```python
from build123d import *

# Parameters (mm, degrees)
SKETCH_1_W          = 20
SKETCH_1_H          = 20
SKETCH_1_R          = 1
EXTRUDE_1_DEPTH     = 28
EXTRUDE_2_DEPTH     = 1.6
SKETCH_3_R          = 2
EXTRUDE_3_DEPTH     = 10.4
CUT_EXTRUDE_START   = -7
CUT_EXTRUDE_4_DEPTH = 7


with BuildPart() as part:
    # 草图1 → 凸台-拉伸1 (new body)
    with BuildSketch(Plane(origin=(0, 0, 0), x_dir=(1, 0, 0), z_dir=(0, 1, 0))):
        with Locations((10, 10)):
            Rectangle(SKETCH_1_W, SKETCH_1_H)
        with Locations(Location((17.7, 2.3, 0), (0, 0, 270))):
            Circle(SKETCH_1_R, mode=Mode.SUBTRACT)
        with Locations(Location((17.7, 17.7, 0), (0, 0, 270))):
            Circle(SKETCH_1_R, mode=Mode.SUBTRACT)
        with Locations(Location((2.3, 17.7, 0), (0, 0, 270))):
            Circle(SKETCH_1_R, mode=Mode.SUBTRACT)
        with Locations(Location((2.3, 2.3, 0), (0, 0, 270))):
            Circle(SKETCH_1_R, mode=Mode.SUBTRACT)
    extrude(amount=EXTRUDE_1_DEPTH)

    # 草图2 → 凸台-拉伸2 (add)
    with BuildSketch(Plane(origin=(0, 28, 0), x_dir=(1, 0, 0), z_dir=(0, 1, 0))):
        with BuildLine():
            ThreePointArc((2, 10), (10, 2), (18, 10))
            Line((18, 10), (2, 10))
        make_face()
        with BuildLine():
            Line((2, 10), (18, 10))
            ThreePointArc((18, 10), (10, 18), (2, 10))
        make_face()
    extrude(amount=EXTRUDE_2_DEPTH)

    # 草图3 → 凸台-拉伸3 (add)
    with BuildSketch(Plane(origin=(0, 29.6, 0), x_dir=(1, 0, 0), z_dir=(0, 1, 0))):
        with Locations(Location((10, 10, 0), (0, 0, 270))):
            Circle(SKETCH_3_R)
    extrude(amount=EXTRUDE_3_DEPTH)

    # 草图4 → 切除-拉伸4 (cut)
    with BuildSketch(Plane(origin=(0, 40, 0), x_dir=(1, 0, 0), z_dir=(0, 1, 0)).offset(CUT_EXTRUDE_START)):
        with BuildLine():
            Line((11.501110762, 11.321615103), (11.501110762, 10))
            Line((11.501110762, 10), (11.501110762, 8.678384897))
            ThreePointArc((11.501110762, 8.678384897), (11.871125533, 9.293679083), (12, 10))
            ThreePointArc((12, 10), (11.871125533, 10.706320917), (11.501110762, 11.321615103))
        make_face()
    extrude(amount=CUT_EXTRUDE_4_DEPTH, mode=Mode.SUBTRACT)


solid = part.part
```
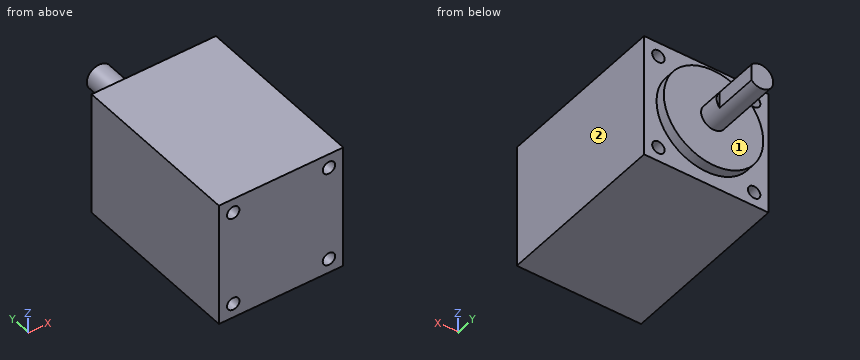
Check sheet for the modelled part. Datum: model origin and axes. Units: mm. Face numbers are marked on the shaded views. A direction names the side the tool comes from. Give positions to 0.01 mm unless a question says otherwise; leave off trailing zeros. Loops run counter-clockwise (first coordinate to the right, second up) from the corner with the lowest first, then second, coordinate; pieces in that order, holes last. Notation, with made-up numbers: M 31,41 L 90,41 A16 cw 90,47 Z; hole C -29,35 d4. An arc over 180 degrees is marked long. Answer in a Markdown table with one row per item.
1) Thickness scan on line 1 (X direction, y = 13, z = -17.7); line 2 (Y direction, x = 4.75, z = -13.5); line 3 (Y direction, x = 2.25, z = -5). Record the ranges inside material, lowest first.
Solutions:
| item | result |
|---|---|
| line 1 | x = 0 to 1.3, 3.3 to 16.7, 18.7 to 20 |
| line 2 | y = 0 to 29.6 |
| line 3 | y = 0 to 28 |
2) Cross-section at D-D (z = -15.25). Enter the section's corners in (x, y), plus the area to 3 significant figures.
Solutions:
| item | result |
|---|---|
| outline | M 0,0 L 20,0 L 20,28 L 16.04,28 L 16.04,29.6 L 3.96,29.6 L 3.96,28 L 0,28 Z |
| area | 579 mm^2 |
3) Cross-section at A-A (y = 22.5). Enter the section's corners in (x, z).
Solutions:
| item | result |
|---|---|
| outline | M 0,-20 L 20,-20 L 20,0 L 0,0 Z; hole C 2.3,-17.7 d2; hole C 2.3,-2.3 d2; hole C 17.7,-17.7 d2; hole C 17.7,-2.3 d2 |
4) Cross-section at B-B (z = -10). Enter the section's corners in (x, y).
Solutions:
| item | result |
|---|---|
| outline | M 0,0 L 20,0 L 20,28 L 18,28 L 18,29.6 L 12,29.6 L 12,33 L 11.5,33 L 11.5,40 L 8,40 L 8,29.6 L 2,29.6 L 2,28 L 0,28 Z |
5) Tool access check on the marked faces 1 and 2. Record the directions out of +Z, -Z, +X, -X, +Y, -Y that give a thin tool (end or side, any length) a straight path to the whole face; none if there is none.
Solutions:
| item | result |
|---|---|
| face 1 | +Y |
| face 2 | +Z, -Z, +X, +Y, -Y |
6) Cross-section at C-C (y = 34). Enter the section's corners in (x, z).
Solutions:
| item | result |
|---|---|
| outline | M 11.5,-11.32 L 11.5,-8.68 A2 ccw long Z |
7) Depth check by flat-ended pin: pin 1 (2 mm diameter, centred on y = 35.5, z = -10.5, fed in from +X); pin 2 (2 mm diameter, centred on y = 31, z = -6.5, fed in from -X); pin 3 (3 mm diameter, centred on x = 11, y = 33.5, fed in from -Z); pin 4 (6 mm diameter, centred on x = 8.5, z = -16, fed in from +Y). Enter the tip coordinate at first touch or a pass-through.
Solutions:
| item | result |
|---|---|
| pin 1 | stops at x = 11.5 |
| pin 2 | passes through |
| pin 3 | stops at z = -12 |
| pin 4 | stops at y = 29.6 |
